from build123d import *

# Parameters (mm, degrees)
SKETCH_1_W          = 130
SKETCH_1_H          = 130
EXTRUDE_1_DEPTH     = 5
CUT_EXTRUDE_2_REACH = 94.06
SKETCH_5_R          = 45
FILLET_1_R          = 10
CUT_EXTRUDE_3_DEPTH = 10
SKETCH_7_R          = 2.5
CUT_EXTRUDE_4_DEPTH = 93.059763198


with BuildPart() as part:
    # 草图1 → 凸台-拉伸1 (new body)
    with BuildSketch(Plane.XY):
        Rectangle(SKETCH_1_W, SKETCH_1_H)
    extrude(amount=EXTRUDE_1_DEPTH)

    # 草图5 → 切除-拉伸2 (cut, up to next)
    with BuildSketch(Plane(origin=(0, 0, 0), x_dir=(-1, 0, 0), z_dir=(0, 0, -1)), mode=Mode.PRIVATE) as cut_extrude_2_sk1:
        Circle(SKETCH_5_R)
    cut_extrude_2_tool1 = extrude(cut_extrude_2_sk1.sketch, amount=-CUT_EXTRUDE_2_REACH, mode=Mode.PRIVATE) & part.part
    add(cut_extrude_2_tool1.solids().sort_by_distance((0, 0, 0))[0], mode=Mode.SUBTRACT)

    # 圆角1
    fillet_1_edges = [part.edges().sort_by_distance(p)[0] for p in [
        (65, -65, 2.5),
        (-65, -65, 2.5),
        (-65, 65, 2.5),
        (65, 65, 2.5),
    ]]
    fillet(fillet_1_edges, radius=FILLET_1_R)

    # 草图6 → 切除-拉伸3 (cut)
    with BuildSketch(Plane(origin=(0, 0, 0), x_dir=(-1, 0, 0), z_dir=(0, 0, -1))):
        with BuildLine():
            ThreePointArc((39.675797976, 38.449883679), (35.787189387, 38.510902038), (35.726171029, 34.622293449))
            ThreePointArc((35.726171029, 34.622293449), (39.614779618, 34.56127509), (39.675797976, 38.449883679))
        make_face()
        with BuildLine():
            ThreePointArc((54.468351255, 1.090089298), (50.579742665, 1.151107656), (50.518724307, -2.737500933))
            ThreePointArc((50.518724307, -2.737500933), (54.407332896, -2.798519291), (54.468351255, 1.090089298))
        make_face()
        with BuildLine():
            ThreePointArc((38.510902038, -35.787189387), (34.622293449, -35.726171029), (34.56127509, -39.614779618))
            ThreePointArc((34.56127509, -39.614779618), (38.449883679, -39.675797976), (38.510902038, -35.787189387))
        make_face()
        with BuildLine():
            ThreePointArc((1.151107656, -50.579742665), (-2.737500933, -50.518724307), (-2.798519291, -54.407332896))
            ThreePointArc((-2.798519291, -54.407332896), (1.090089298, -54.468351255), (1.151107656, -50.579742665))
        make_face()
        with BuildLine():
            ThreePointArc((-35.726171029, -34.622293449), (-39.614779618, -34.56127509), (-39.675797976, -38.449883679))
            ThreePointArc((-39.675797976, -38.449883679), (-35.787189387, -38.510902038), (-35.726171029, -34.622293449))
        make_face()
        with BuildLine():
            ThreePointArc((-50.518724307, 2.737500933), (-54.407332896, 2.798519291), (-54.468351255, -1.090089298))
            ThreePointArc((-54.468351255, -1.090089298), (-50.579742665, -1.151107656), (-50.518724307, 2.737500933))
        make_face()
        with BuildLine():
            ThreePointArc((-34.56127509, 39.614779618), (-38.449883679, 39.675797976), (-38.510902038, 35.787189387))
            ThreePointArc((-38.510902038, 35.787189387), (-34.622293449, 35.726171029), (-34.56127509, 39.614779618))
        make_face()
        with BuildLine():
            ThreePointArc((2.798519291, 54.407332896), (-1.090089298, 54.468351255), (-1.151107656, 50.579742665))
            ThreePointArc((-1.151107656, 50.579742665), (2.737500933, 50.518724307), (2.798519291, 54.407332896))
        make_face()
    extrude(amount=-CUT_EXTRUDE_3_DEPTH, mode=Mode.SUBTRACT)

    # 草图7 → 切除-拉伸4 (cut, through all)
    with BuildSketch(Plane.XY.offset(5)):
        with Locations((-45, 45)):
            Circle(SKETCH_7_R)
        with Locations((45, 45)):
            Circle(SKETCH_7_R)
        with Locations((45, -45)):
            Circle(SKETCH_7_R)
        with Locations((-45, -45)):
            Circle(SKETCH_7_R)
    extrude(amount=-CUT_EXTRUDE_4_DEPTH, mode=Mode.SUBTRACT)


solid = part.part
Verification items for the finished model (mm, model axes). Give positions to 0.01 mm unless a question says otherwise; leave off trailing zeros. Loops run counter-clockwise (first coordinate to the right, second up) from the corner with the lowest first, then second, coordinate; pieces in that order, holes last.
1) Sectioned sample at C-C, the plane x = -19.5. Enter the section's corners in (y, z).
2) Sectioned sample at A-A, the plane y = 12.5. Enter the section's corners in (x, z), then the cut area to 3 significant figures.
3) Draft check along X on faces 1 (the cylindrical face through (-42.69, 44.04, 2.54)), 2 (the flat face through (-1, -65, 2)), 3 (the cylindrical face through (61.99, -62.15, 2.54)). Enter one of: pulls with the +X half, pulls with the -X half, needs draft (parallel to the pull), parting line crosses it, or undercut.
4) Thickness scan on line 1 along Y through (x, z) = (-38, 3.05); line 2 along Y through (x, z) = (39, 2.95); line 3 along Y through (x, z) = (-40, 4.6). Record the ranges inside material, lowest first.
5) Sectioned sample at B-B, the plane z = 3.2. Count the separate pieces of the cut face and the enclosed holes in it, then the cut area to 3 significant figures.
Answers:
1. outline: (-65, 0) - (-40.56, 0) - (-40.56, 5) - (-65, 5) - close; (40.56, 0) - (65, 0) - (65, 5) - (40.56, 5) - close
2. outline: (-65, 0) - (-43.23, 0) - (-43.23, 5) - (-65, 5) - close; (43.23, 0) - (65, 0) - (65, 5) - (43.23, 5) - close
2. area: 218 mm2
3. face 1: undercut
3. face 2: needs draft
3. face 3: pulls with the +X half
4. line 1: y = -65 to -40.03, -35.37 to -24.1, 24.1 to 33.8, 39.27 to 65
4. line 2: y = -65 to -38.96, -34.11 to -22.45, 22.45 to 36.48, 38.92 to 65
4. line 3: y = -65 to -20.62, 20.62 to 35.03, 38.05 to 65
5. separate pieces: 1
5. enclosed holes: 13
5. area: 10,200 mm2
